from build123d import *

# Parameters (mm, degrees)
SKETCH1_R               = 22.225
BOSS_EXTRUDE1_DEPTH     = 21
SKETCH3_R               = 10
CUT_EXTRUDE1_DEPTH      = 7
BOSS_EXTRUDE2_DEPTH     = 71
SKETCH5_W               = 150
SKETCH5_H               = 180
CUT_EXTRUDE2_DEPTH      = 72
SKETCH6_RX              = 48.683272643
SKETCH6_RY              = 26.408297454
BOSS_EXTRUDE3_DEPTH     = 8
BOSS_EXTRUDE4_OUTLINE_W = 150.225
BOSS_EXTRUDE4_OUTLINE_H = 1
BOSS_EXTRUDE4_DEPTH     = 21


# Read off the part's stored shape, not the designer's step: Boss-Extrude4
with BuildPart() as part:
    # Sketch1 → Boss-Extrude1 (new body)
    with BuildSketch(Plane(origin=(0, 0, 0), x_dir=(1, 0, 0), z_dir=(0, 1, 0))):
        with Locations(Location((0, 0, 0), (0, 0, 90))):
            Circle(SKETCH1_R)
    extrude(amount=BOSS_EXTRUDE1_DEPTH)

    # Sketch3 → Cut-Extrude1 (cut)
    with BuildSketch(Plane.XZ):
        with Locations(Location((0, 0, 0), (0, 0, 270))):
            Circle(SKETCH3_R)
    extrude(amount=-CUT_EXTRUDE1_DEPTH, mode=Mode.SUBTRACT)

    # Sketch4 → Boss-Extrude2 (add)
    with BuildSketch(Plane(origin=(0, 21, 0), x_dir=(1, 0, 0), z_dir=(0, 1, 0))):
        Polygon((0, 0), (-4.5, 0), (-4.5, 2.598076211), (-21.098752445, -6.985217981), (-16.598752445, -14.779446615), (0, -5.196152423), (-2.25, -3.897114317), align=None)
        Polygon((4.5, 0), (0, 0), (2.25, -3.897114317), (0, -5.196152423), (16.598752445, -14.779446615), (21.098752445, -6.985217981), (4.5, 2.598076211), align=None)
        Polygon((-2.25, 3.897114317), (0, 0), (2.25, 3.897114317), (4.5, 2.598076211), (4.5, 21.764664597), (-4.5, 21.764664597), (-4.5, 2.598076211), align=None)
        Polygon((2.25, -3.897114317), (0, 0), (-2.25, -3.897114317), (0, -5.196152423), align=None)
        Polygon((-4.5, 2.598076211), (-4.5, 0), (0, 0), (-2.25, 3.897114317), align=None)
        Polygon((2.25, 3.897114317), (0, 0), (4.5, 0), (4.5, 2.598076211), align=None)
    extrude(amount=BOSS_EXTRUDE2_DEPTH)

    # Sketch5 → Cut-Extrude2 (cut)
    with BuildSketch(Plane(origin=(0, 35.117667702, 35.117667702), x_dir=(-1, 0, 0), z_dir=(0, -0.7071067811865488, -0.7071067811865464))):
        Rectangle(SKETCH5_W, SKETCH5_H)
    extrude(amount=-CUT_EXTRUDE2_DEPTH, mode=Mode.SUBTRACT)

    # Sketch6 → Boss-Extrude3 (add)
    with BuildSketch(Plane(origin=(0, 35.117667702, 35.117667702), x_dir=(1, 0, 0), z_dir=(0, 0.7071067811865487, 0.7071067811865464))):
        with Locations(Location((0, 42.315412714), (0, 0, 90))):
            Ellipse(SKETCH6_RX, SKETCH6_RY)
    extrude(amount=BOSS_EXTRUDE3_DEPTH)

    # Boss-Extrude4 outline → Boss-Extrude4 (add)
    with BuildSketch(Plane(origin=(0, 0, 0), x_dir=(1, 0, 0), z_dir=(0, 1, 0))):
        with Locations((-97.1125, 0)):
            Rectangle(BOSS_EXTRUDE4_OUTLINE_W, BOSS_EXTRUDE4_OUTLINE_H)
    extrude(amount=BOSS_EXTRUDE4_DEPTH)


solid = part.part
Design review of the part built by this model. Coordinates are the model's own, in mm. A direction names the side the tool comes from. Round coordinates to 2 decimals unless told otherwise and drop trailing zeros. Order: outer loops, then holes, each group sorted by start corner. A loop starts at its lowest first (then second) coordinate and runs counter-clockwise, first axis right, second up.
1) Machinability: for faces 1 (the flat face through (-19, 21, 11)), 2 (the flat face through (8.18, 42.71, 9.92)), 3 (the flat face through (0, 21, 14)), which of the approach directions +Z, -Z, +X, -X, +Y, -Y give a long, thin tool a straight path to every point of the face, cutting with its end or side? Answer none if there is none.
The answers:
face 1: +Z, -X
face 2: none
face 3: +Z
2) Draft analysis for pull direction Y (two halves, no side actions). For faces 4 (the flat face through (-98, 10, 0.5)), 5 (the flat face through (-18, 0, -2)), 6 (the flat face through (-18.88, 41.83, 10.83)), state which applies: released by +Y, released by -Y, zero draft, split by the parting line, or undercut.
The answers:
face 4: zero draft
face 5: released by -Y
face 6: undercut
3) Clearance check with flat-ended pins moving along their axes: pin 1 Ø12 at (y, z) = (34.5, 34.5) entering from -X; pin 2 Ø17 at (x, y) = (-121, 6) entering from +Z; pin 3 Ø6.5 at (x, y) = (-94, 13) entering from -Z. State where each tip first meets the part, or that it passes through.
The answers:
pin 1: stops at x = -17.55
pin 2: stops at z = 0.5
pin 3: stops at z = -0.5
4) Consider section B-B (x = -125). State the section outline as (y, z) points.
The answers:
outline: (0, -0.5) - (21, -0.5) - (21, 0.5) - (0, 0.5) - close
5) For L1, parallel to X at y = 4, z = 0 (3 decimals); L2, parallel to Z at x = -154.5, y = 7; L3, parallel to X at y = 18, z = -1, list the stretches that pass through material, from the lowest coordinate up.
The answers:
L1: x = -172.225 to -10, 10 to 22.225
L2: z = -0.5 to 0.5
L3: x = -22.2 to 22.2
6) Consider section A-A (y = 26.5). State the section outline as (x, z) points.
The answers:
outline: (-21.1, 6.99) - (-4.5, -2.6) - (-4.5, -21.76) - (4.5, -21.76) - (4.5, -2.6) - (21.1, 6.99) - (16.6, 14.78) - (0, 5.2) - (-16.6, 14.78) - close
